Can you work these out from the model? Positions are in its coordinate system, mm. Round coordinates to 2 decimals unless told otherwise and drop trailing zeros. Loops run counter-clockwise (first coordinate to the right, second up) from the corner with the lowest first, then second, coordinate; pieces in that order, holes last. Notation, with made-up numbers: (-13, 66.25) -> (-7, 66.25) arc R20 ccw to (-7, 84.25) -> close; hole circle Ø5 at (29, -15). An arc over 180 degrees is marked (long way). Answer as a JSON object with one key per item and string values.
```python
from build123d import *

# Parameters (mm, degrees)
SKETCH_1_R      = 2
SKETCH_1_R_2    = 1.5
EXTRUDE_1_DEPTH = 6
SKETCH_1_2_R    = 1.5
EXTRUDE_2_DEPTH = 200


with BuildPart() as part:
    # 草图1 → 凸台-拉伸1 (new body)
    with BuildSketch(Plane.XY):
        with BuildLine():
            Line((-6.403124237, -20), (6.403124237, -20))
            ThreePointArc((6.403124237, -20), (13.429663608, -16.144476931), (18.5, -9.937303457))
            Line((18.5, -9.937303457), (18.5, 9.937303457))
            ThreePointArc((18.5, 9.937303457), (0, 21), (-18.5, 9.937303457))
            Line((-18.5, 9.937303457), (-18.5, -9.937303457))
            ThreePointArc((-18.5, -9.937303457), (-13.429663608, -16.144476931), (-6.403124237, -20))
        make_face()
        Circle(SKETCH_1_R, mode=Mode.SUBTRACT)
        with Locations((0, 16)):
            Circle(SKETCH_1_R_2, mode=Mode.SUBTRACT)
    extrude(amount=-EXTRUDE_1_DEPTH)

    # 草图1<2> → 凸台-拉伸2 (add)
    with BuildSketch(Plane.XY):
        with Locations((0, 16)):
            Circle(SKETCH_1_2_R)
    extrude(amount=-EXTRUDE_2_DEPTH)


solid = part.part
```
Q1. I want a section at D-D, the plane x = -4.5. Write out the boundary of the cut face in (y, z).
Determined:
{"outline": "(-20, -6) -> (20.51, -6) -> (20.51, 0) -> (-20, 0) -> close"}
Q2. We'd pull the mould along Y, two halves only. Please class faces 1 (the flat face through (4, 1, 0)), 2 (the flat face through (0, -20, -3)), 3 (the cylindrical face through (0, -2, -3)): pulls with the +Y half, pulls with the -Y half, needs draft (parallel to the pull), parting line crosses it, or undercut.
Determined:
{"face 1": "needs draft", "face 2": "pulls with the -Y half", "face 3": "undercut"}
Q3. I want a section at B-B, the plane z = -180.5. Write out the boundary of the cut face in (x, y).
Determined:
{"outline": "circle Ø3 at (0, 16)"}
Q4. If I drill on L1, parallel to Z at x = 6, y = 12.5; L2, parallel to Y at x = 1, z = -128.5, over which ranges is the centre line in solid material (lowest first)? Write a range as [from, to].
Determined:
{"L1": "[-6, 0]", "L2": "[14.88, 17.12]"}
Q5. I want a section at A-A, the plane y = 0. Write out the boundary of the cut face in (x, z).
Determined:
{"outline": "(-18.5, -6) -> (-2, -6) -> (-2, 0) -> (-18.5, 0) -> close; (2, -6) -> (18.5, -6) -> (18.5, 0) -> (2, 0) -> close"}
Q6. I'm going to push flat-ended pins straight in: pin 1 (12 mm diameter, centred on y = 11, z = -20, fed in from +X); pin 2 (1 mm diameter, centred on x = 12.5, y = 15, fed in from -Z); pin 3 (8 mm diameter, centred on x = -14, y = 0.5, fed in from +Z); pin 4 (3 mm diameter, centred on x = 0, y = 0, fed in from -Z). Where does each tip first touch, or does it pass through?
Determined:
{"pin 1": "x = 1.5", "pin 2": "z = -6", "pin 3": "z = 0", "pin 4": "through"}
Q7. I want a section at C-C, the plane x = 16. Write out the boundary of the cut face in (y, z).
Determined:
{"outline": "(-13.6, -6) -> (13.6, -6) -> (13.6, 0) -> (-13.6, 0) -> close"}
